```python
from build123d import *

# Parameters (mm, degrees)
CROQUIS1_R              = 7.25
SALIENTE_EXTRUIR1_DEPTH = 30
CROQUIS2_R              = 1.4
CORTAR_EXTRUIR1_DEPTH   = 41.332305418
CHAFL_N2_SIZE           = 0.85
CHAFL_N3_SIZE           = 0.7
CHAFL_N4_SIZE           = 0.5


with BuildPart() as part:
    # Croquis1 → Saliente-Extruir1 (new body)
    with BuildSketch(Plane.XY):
        Polygon((-15.39, 16.407843258), (-15.39, 5.26761363), (-16.85, 4.396751988), (-16.85, -0.603248012), (-16.46109127, -0.992156742), (-7.275, -0.992156742), (-6.15, 0), (6.15, 0), (7.275, -0.992156742), (16.46109127, -0.992156742), (16.85, -0.603248012), (16.85, 4.396751988), (15.39, 5.26761363), (15.39, 16.407843258), (8.4, 16.407843258), (4.5, 20.05), (-4.5, 20.05), (-8.4, 16.407843258), align=None)
        with Locations((0, 9.55)):
            Circle(CROQUIS1_R, mode=Mode.SUBTRACT)
    extrude(amount=-SALIENTE_EXTRUIR1_DEPTH)

    # Croquis2 → Cortar-Extruir1 (cut, through all)
    with BuildSketch(Plane.XZ.offset(0.992156742)):
        with Locations((-12.95, -5.4)):
            Circle(CROQUIS2_R)
        with Locations(Location((-12.95, -24.6, 0), (0, 0, 270))):
            Circle(CROQUIS2_R)
        with Locations((12.95, -24.6)):
            Circle(CROQUIS2_R)
        with Locations(Location((12.95, -5.4, 0), (0, 0, 90))):
            Circle(CROQUIS2_R)
    extrude(amount=-CORTAR_EXTRUIR1_DEPTH, mode=Mode.SUBTRACT)

    # Chaflán2
    chafl_n2_edges = [part.edges().sort_by_distance(p)[0] for p in [
        (12.95, -0.992156742, -6.8),
        (11.55, -0.992156742, -24.6),
        (-12.95, -0.992156742, -23.2),
        (-14.35, -0.992156742, -5.4),
    ]]
    chamfer(chafl_n2_edges, length=CHAFL_N2_SIZE)

    # Chaflán3
    chafl_n3_edges = [part.edges().sort_by_distance(p)[0] for p in [
        (-12.95, 16.407843258, -23.2),
        (-14.35, 16.407843258, -5.4),
    ]]
    chamfer(chafl_n3_edges, length=CHAFL_N3_SIZE)

    # Chaflán4
    chafl_n4_edges = [part.edges().sort_by_distance(p)[0] for p in [
        (12.95, 16.407843258, -6.8),
        (11.55, 16.407843258, -24.6),
    ]]
    chamfer(chafl_n4_edges, length=CHAFL_N4_SIZE)


solid = part.part
```
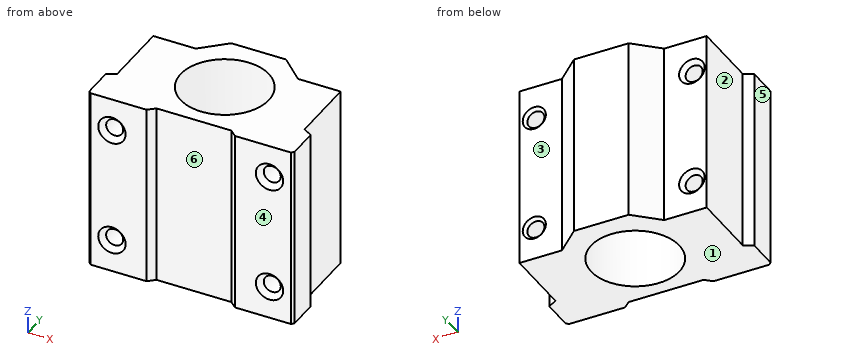
Work out the finished part from the listing and answer in its coordinate system (mm). Face numbers are marked on the shaded views. A direction names the side the tool comes from. Give positions to 0.01 mm unless a question says otherwise; leave off trailing zeros. Order: outer loops, then holes, each group sorted by start corner. A loop starts at its lowest first (then second) coordinate and runs counter-clockwise, first axis right, second up. Notation, with made-up numbers: M 77.25,39 L 90.25,39 A20 cw 90.25,50 Z; hole C 66,14 d11. An arc over 180 degrees is marked long. Return JSON: item names as keys, results as strings.
1) A tool of negligible diameter and unlimited length cuts with its end or side. For the marked faces 1, 2 and 3, from which of +Z, -Z, +X, -X, +Y, -Y can it reach the whole face along a straight path? Write none if from no direction.
Resolved:
{"face 1": "-Z, +X, -X, +Y, -Y", "face 2": "+Z, -Z, -X, +Y", "face 3": "+Z, -Z, +X, +Y"}
2) Section A-A, the plane x = -12.95 is taken. Write down the section's boundary in (y, z), plus the area to 3 significant figures.
Resolved:
{"outline": "M -0.99,-30 L 16.41,-30 L 16.41,-26.7 L 15.71,-26 L -0.14,-26 L -0.99,-26.85 Z; M -0.99,-22.35 L -0.14,-23.2 L 15.71,-23.2 L 16.41,-22.5 L 16.41,-7.5 L 15.71,-6.8 L -0.14,-6.8 L -0.99,-7.65 Z; M -0.99,-3.15 L -0.14,-4 L 15.71,-4 L 16.41,-3.3 L 16.41,0 L -0.99,0 Z", "area": "422 mm^2"}
3) Straight lines are drawn through the part: line 1 along Z through (x, y) = (-13, 6.5); line 2 along X through (y, z) = (16.25, -25.75); line 3 along X through (y, z) = (0.5, -23.5). For each, find the intervals that lie inside material, in ascending order. Write a range as [from, to].
Resolved:
{"line 1": "[-30, -26], [-23.2, -6.8], [-4, 0]", "line 2": "[-15.39, -14.52], [-11.38, -2.77], [2.77, 11.64], [14.26, 15.39]", "line 3": "[-16.85, -13.82], [-12.08, 12.08], [13.82, 16.85]"}
4) For a pull along X with two mould halves and no side action, classify the marked faces 4, 5 and 6 as +X half, -X half, draft (parallel to the pull), parting line (faces both ways), or undercut.
Resolved:
{"face 4": "draft", "face 5": "-X half", "face 6": "undercut"}
5) Section D-D, the plane x = 0 is taken. Write down the section's boundary in (y, z), plus the area to 4 significant figures.
Resolved:
{"outline": "M 0,-30 L 2.3,-30 L 2.3,0 L 0,0 Z; M 16.8,-30 L 20.05,-30 L 20.05,0 L 16.8,0 Z", "area": "166.5 mm^2"}
6) Section C-C, the plane z = -13.25 is taken. Write down the section's boundary in (x, y) (3 decimals).
Resolved:
{"outline": "M -16.85,-0.603 L -16.461,-0.992 L -7.275,-0.992 L -6.15,0 L 6.15,0 L 7.275,-0.992 L 16.461,-0.992 L 16.85,-0.603 L 16.85,4.397 L 15.39,5.268 L 15.39,16.408 L 8.4,16.408 L 4.5,20.05 L -4.5,20.05 L -8.4,16.408 L -15.39,16.408 L -15.39,5.268 L -16.85,4.397 Z; hole C 0,9.55 d14.5"}
7) Section B-B, the plane y = 9.55 is taken. Write down the section's boundary in (x, z).
Resolved:
{"outline": "M -15.39,-30 L -7.25,-30 L -7.25,0 L -15.39,0 Z; M 7.25,-30 L 15.39,-30 L 15.39,0 L 7.25,0 Z; hole C -12.95,-24.6 d2.8; hole C -12.95,-5.4 d2.8; hole C 12.95,-24.6 d2.8; hole C 12.95,-5.4 d2.8"}
8) Each of these flat-tipped pins is pushed along its axis until it touches: pin 1 (10 mm diameter, centred on y = 13.5, z = -25.5, fed in from -X); pin 2 (3 mm diameter, centred on x = 12.95, z = -5.4, fed in from -Y); pin 3 (2 mm diameter, centred on x = 12.95, z = -24.6, fed in from +Y); pin 4 (3.5 mm diameter, centred on x = -12.5, z = -14.5, fed in from +Y). Where does it stop, or does it pass through?
Resolved:
{"pin 1": "x = -15.39", "pin 2": "y = -0.24", "pin 3": "through", "pin 4": "y = 16.41"}
